Autodesk Inventor part; units mm, degrees
ref_plane "YZ Plane" through (0, 0, 0) normal (1, 0, 0) x (0, 1, 0)
ref_plane "XZ Plane" through (0, 0, 0) normal (0, 1, 0) x (-1, 0, 0)
ref_plane "XY Plane" through (0, 0, 0) normal (0, 0, 1) x (1, 0, 0)
sketch "Эскиз1" plane through (0, 0, 0) normal (0, 0, 1) x (1, 0, 0)
  circle A0 centre (0, 0) radius 10
  line L0 (-3.8095, 3.8095) -> (3.8095, 3.8095)
  line L1 (3.8095, 3.8095) -> (3.8095, -3.8095)
  line L2 (3.8095, -3.8095) -> (-3.8095, -3.8095)
  line L3 (-3.8095, -3.8095) -> (-3.8095, 3.8095)
  line L4 (-3.8095, 3.8095) -> (3.8095, -3.8095) construction
  line L5 (3.8095, 3.8095) -> (-3.8095, -3.8095) construction
  dimension "d0" = 20
extrude "Выдавливание1" add sketch "Эскиз1" along normal blind 36
sketch "Эскиз2" plane through (0, 0, 36) normal (0, 0, 1) x (1, 0, 0)
  line L0 (-3.8095, 3.8095) -> (3.8095, 3.8095)
  circle A0 centre (0, 0) radius 10
  line L1 (9.8151, 1.914) -> (5.5, 1.0725)
  line L2 (5.5, -1.0775) -> (9.8135, -1.9225)
  line L3 (5.5, 0) -> (5.5, 1.0725)
  line L4 (5.5, 1.0725) -> (5.5, -1.0775)
  line L5 (5.587, 8.2937) -> (3.1307, 4.6475)
  line L6 (4.651, 3.1272) -> (8.2986, 5.5797)
  line L7 (3.8891, 3.8891) -> (3.1307, 4.6475)
  line L8 (3.1307, 4.6475) -> (4.651, 3.1272)
  line L9 (-1.914, 9.8151) -> (-1.0725, 5.5)
  line L10 (1.0775, 5.5) -> (1.9225, 9.8135)
  line L11 (0, 5.5) -> (-1.0725, 5.5)
  line L12 (-1.0725, 5.5) -> (1.0775, 5.5)
  line L13 (-8.2937, 5.587) -> (-4.6475, 3.1307)
  line L14 (-3.1272, 4.651) -> (-5.5797, 8.2986)
  line L15 (-3.8891, 3.8891) -> (-4.6475, 3.1307)
  line L16 (-4.6475, 3.1307) -> (-3.1272, 4.651)
  line L17 (-9.8151, -1.914) -> (-5.5, -1.0725)
  line L18 (-5.5, 1.0775) -> (-9.8135, 1.9225)
  line L19 (-5.5, 0) -> (-5.5, -1.0725)
  line L20 (-5.5, -1.0725) -> (-5.5, 1.0775)
  line L21 (-5.587, -8.2937) -> (-3.1307, -4.6475)
  line L22 (-4.651, -3.1272) -> (-8.2986, -5.5797)
  line L23 (-3.8891, -3.8891) -> (-3.1307, -4.6475)
  line L24 (-3.1307, -4.6475) -> (-4.651, -3.1272)
  line L25 (1.914, -9.8151) -> (1.0725, -5.5)
  line L26 (-1.0775, -5.5) -> (-1.9225, -9.8135)
  line L27 (0, -5.5) -> (1.0725, -5.5)
  line L28 (1.0725, -5.5) -> (-1.0775, -5.5)
  line L29 (8.2937, -5.587) -> (4.6475, -3.1307)
  line L30 (3.1272, -4.651) -> (5.5797, -8.2986)
  line L31 (3.8891, -3.8891) -> (4.6475, -3.1307)
  line L32 (4.6475, -3.1307) -> (3.1272, -4.651)
  dimension "d36" = 360
extrude "Выдавливание2" add sketch "Эскиз2" along normal blind 3 contours A0 L2 L4 L3 L1 | L6 L8 L7 L5 A0 | A0 L30 L32 L31 L29 | L10 L12 L11 L9 A0 | A0 L26 L28 L27 L25 | L14 L16 L15 L13 A0 | A0 L22 L24 L23 L21 | L18 L20 L19 L17 A0
chamfer "Фаска1" distance 2 angle 10 1 edges at (4.3588, 6.4706, 39) measured on face at (4.7682, 7.0783, 37)
chamfer "Фаска2" distance 2 angle 10 1 edges at (6.4748, 4.3535, 39) measured on face at (5.8669, 3.9447, 37)
chamfer "Фаска3" distance 2 angle 10 1 edges at (7.6576, 1.4932, 39) measured on face at (8.3768, 1.6335, 37)
chamfer "Фаска4" distance 2 angle 10 1 edges at (7.6567, -1.5, 39) measured on face at (6.9378, -1.3592, 37)
chamfer "Фаска5" distance 2 angle 10 1 edges at (6.4706, -4.3588, 39) measured on face at (7.0783, -4.7682, 37)
chamfer "Фаска6" distance 2 angle 10 1 edges at (4.3535, -6.4748, 39) measured on face at (3.9447, -5.8669, 37)
chamfer "Фаска7" distance 2 angle 10 1 edges at (-1.5, -7.6567, 39) measured on face at (-1.3592, -6.9378, 37)
chamfer "Фаска8" distance 2 angle 10 1 edges at (1.4932, -7.6576, 39) measured on face at (1.6335, -8.3768, 37)
chamfer "Фаска9" distance 2 angle 10 1 edges at (-6.4748, -4.3535, 39) measured on face at (-5.8669, -3.9447, 37)
chamfer "Фаска10" distance 2 angle 10 1 edges at (-4.3588, -6.4706, 39) measured on face at (-4.7682, -7.0783, 37)
chamfer "Фаска11" distance 2 angle 10 1 edges at (-7.6567, 1.5, 39) measured on face at (-6.9378, 1.3592, 37)
chamfer "Фаска12" distance 2 angle 10 1 edges at (-7.6576, -1.4932, 39) measured on face at (-8.3768, -1.6335, 37)
chamfer "Фаска13" distance 2 angle 10 1 edges at (-4.3535, 6.4748, 39) measured on face at (-3.9447, 5.8669, 37)
chamfer "Фаска14" distance 2 angle 10 1 edges at (-6.4706, 4.3588, 39) measured on face at (-7.0783, 4.7682, 37)
chamfer "Фаска15" distance 2 angle 10 1 edges at (1.5, 7.6567, 39) measured on face at (1.3592, 6.9378, 37)
chamfer "Фаска16" distance 2 angle 10 1 edges at (-1.4932, 7.6576, 39) measured on face at (-1.6335, 8.3768, 37)
sketch "Эскиз3" plane through (0, 0, 36) normal (0, 0, 1) x (1, 0, 0)
  point P0 (0, 0)
sketch "Эскиз5" plane through (0, 0, 36) normal (0, 0, 1) x (1, 0, 0)
  point P0 (0, 0)
sketch "Эскиз6" plane through (0, 0, 36) normal (0, 0, 1) x (1, 0, 0)
  line L0 (-1.0725, 5.5) -> (-1.914, 9.8151)
  arc A0 (-1.914, 9.8151) -> (-5.5797, 8.2986) centre (0, 0) ccw
  line L1 (-5.5797, 8.2986) -> (-3.1272, 4.651)
  line L2 (-3.1272, 4.651) -> (-4.6475, 3.1307)
  line L3 (-4.6475, 3.1307) -> (-8.2937, 5.587)
  arc A1 (-8.2937, 5.587) -> (-9.8135, 1.9225) centre (0, 0) ccw
  line L4 (-9.8135, 1.9225) -> (-5.5, 1.0775)
  line L5 (-5.5, 1.0775) -> (-5.5, -1.0725)
  line L6 (-5.5, -1.0725) -> (-9.8151, -1.914)
  arc A2 (-9.8151, -1.914) -> (-8.2986, -5.5797) centre (0, 0) ccw
  line L7 (-8.2986, -5.5797) -> (-4.651, -3.1272)
  line L8 (-4.651, -3.1272) -> (-3.1307, -4.6475)
  line L9 (-3.1307, -4.6475) -> (-5.587, -8.2937)
  arc A3 (-5.587, -8.2937) -> (-1.9225, -9.8135) centre (0, 0) ccw
  line L10 (-1.9225, -9.8135) -> (-1.0775, -5.5)
  line L11 (-1.0775, -5.5) -> (1.0725, -5.5)
  line L12 (1.0725, -5.5) -> (1.914, -9.8151)
  arc A4 (1.914, -9.8151) -> (5.5797, -8.2986) centre (0, 0) ccw
  line L13 (5.5797, -8.2986) -> (3.1272, -4.651)
  line L14 (3.1272, -4.651) -> (4.6475, -3.1307)
  line L15 (4.6475, -3.1307) -> (8.2937, -5.587)
  arc A5 (8.2937, -5.587) -> (9.8135, -1.9225) centre (0, 0) ccw
  line L16 (9.8135, -1.9225) -> (5.5, -1.0775)
  line L17 (5.5, -1.0775) -> (5.5, 1.0725)
  line L18 (5.5, 1.0725) -> (9.8151, 1.914)
  arc A6 (9.8151, 1.914) -> (8.2986, 5.5797) centre (0, 0) ccw
  line L19 (8.2986, 5.5797) -> (4.651, 3.1272)
  line L20 (4.651, 3.1272) -> (3.1307, 4.6475)
  line L21 (3.1307, 4.6475) -> (5.587, 8.2937)
  arc A7 (5.587, 8.2937) -> (1.9225, 9.8135) centre (0, 0) ccw
  line L22 (1.9225, 9.8135) -> (1.0775, 5.5)
  line L23 (1.0775, 5.5) -> (-1.0725, 5.5)
  line L24 (-3.8095, 3.8095) -> (3.8095, 3.8095)
  line L25 (3.8095, 3.8095) -> (3.8095, -3.8095)
  line L26 (3.8095, -3.8095) -> (-3.8095, -3.8095)
  line L27 (-3.8095, -3.8095) -> (-3.8095, 3.8095)
extrude "Выдавливание4" add sketch "Эскиз6" against normal up to surface (36 mm away) contours L24 L25 L26 L27
sketch "Эскиз7" plane through (0, 0, 36) normal (0, 0, 1) x (1, 0, 0)
  line L0 (-5.8493, 2.507) -> (2.507, 5.8493)
  line L1 (2.507, 5.8493) -> (5.8493, -2.507)
  line L2 (5.8493, -2.507) -> (-2.507, -5.8493)
  line L3 (-2.507, -5.8493) -> (-5.8493, 2.507)
  line L4 (-5.8493, 2.507) -> (5.8493, -2.507) construction
  line L5 (2.507, 5.8493) -> (-2.507, -5.8493) construction
  point P0 (0, 0)
  dimension "d95" = 9
  dimension "d96" = 9
extrude "Выдавливание5" cut sketch "Эскиз7" against normal through all
sketch "Эскиз8" plane through (0, 0, 36) normal (0, 0, 1) x (1, 0, 0)
  line L0 (-4.651, -3.1272) -> (-3.1307, -4.6475)
  line L1 (-1.0775, -5.5) -> (1.0725, -5.5)
  line L2 (-3.1307, -4.6475) -> (-1.0775, -5.5)
  line L3 (-1.0775, -5.5) -> (-1.3659, -6.972)
  line L4 (-1.9225, -9.8135) -> (-1.0775, -5.5)
  line L5 (-3.1307, -4.6475) -> (-3.9688, -5.8915)
  line L6 (-3.1307, -4.6475) -> (-5.587, -8.2937)
  line L7 (-3.9688, -5.8915) -> (-1.3659, -6.972)
  line L8 (4.6475, -3.1307) -> (5.8915, -3.9688)
  line L9 (5.5, -1.0775) -> (6.972, -1.3659)
  line L10 (4.6475, -3.1307) -> (5.5, -1.0775)
  line L11 (5.8915, -3.9688) -> (6.972, -1.3659)
  line L12 (3.1307, 4.6475) -> (3.9688, 5.8915)
  line L13 (1.0775, 5.5) -> (1.3659, 6.972)
  line L14 (3.1307, 4.6475) -> (1.0775, 5.5)
  line L15 (3.9688, 5.8915) -> (1.3659, 6.972)
  line L16 (-4.6475, 3.1307) -> (-5.8915, 3.9688)
  line L17 (-5.5, 1.0775) -> (-6.972, 1.3659)
  line L18 (-4.6475, 3.1307) -> (-5.5, 1.0775)
  line L19 (-5.8915, 3.9688) -> (-6.972, 1.3659)
  point P0 (0, 0)
  dimension "d99" = 1.5
  dimension "d100" = 1.5
  dimension "d103" = 360
extrude "Выдавливание6" cut sketch "Эскиз8" against normal through all
sketch "Эскиз9" plane through (0, 0, 36) normal (0, 0, 1) x (1, 0, 0)
  line L0 (-1.3659, -6.972) -> (-1.0775, -5.5)
  line L1 (-1.0775, -5.5) -> (-1, -5)
  line L2 (-3.1307, -4.6475) -> (-3.9688, -5.8915)
  line L3 (-3.1307, -4.6475) -> (-2.4444, -3.6286)
  line L4 (-2.4444, -3.6286) -> (-1, -5)
  line L5 (-3.1307, -4.6475) -> (-1.0775, -5.5)
  line L6 (5.5, -1.0775) -> (5, -1)
  line L7 (4.6475, -3.1307) -> (3.6286, -2.4444)
  line L8 (3.6286, -2.4444) -> (5, -1)
  line L9 (4.6475, -3.1307) -> (5.5, -1.0775)
  line L10 (1.0775, 5.5) -> (1, 5)
  line L11 (3.1307, 4.6475) -> (2.4444, 3.6286)
  line L12 (2.4444, 3.6286) -> (1, 5)
  line L13 (3.1307, 4.6475) -> (1.0775, 5.5)
  line L14 (-5.5, 1.0775) -> (-5, 1)
  line L15 (-4.6475, 3.1307) -> (-3.6286, 2.4444)
  line L16 (-3.6286, 2.4444) -> (-5, 1)
  line L17 (-4.6475, 3.1307) -> (-5.5, 1.0775)
  point P0 (0, 0)
  dimension "d109" = 360
extrude "Выдавливание7" cut sketch "Эскиз9" against normal through all
properties part number "деталь вв"
Check sheet for the modelled part. Datum: model origin and axes. Units: mm. A direction names the side the tool comes from. Round coordinates to 2 decimals unless told otherwise and drop trailing zeros. Order: outer loops, then holes, each group sorted by start corner. A loop starts at its lowest first (then second) coordinate and runs counter-clockwise, first axis right, second up.
(1) Cross-section at C-C, the plane x = -2.5. Enter the section's corners in (y, z).
(2) Cross-section at B-B, the plane x = 0. Enter the section's corners in (y, z), and give its area (3 significant figures).
(3) Scan lines: probe 1 along Y at (x, z) = (8, 36.5); probe 2 along Y at (x, z) = (-2.5, 15); probe 3 along Y at (x, z) = (-3.5, 37). Record each from-to range of solid material in increasing order.
(4) Go/stop test with flat-tipped pins: P1, Ø1.5, axis at y = 7, z = 31.5, coming from the +X side; P2, Ø5, axis at x = -7.5, z = 22.5, coming from the -Y side; P3, Ø8, axis at x = 5, z = 25.5, coming from the -Y side. Record where each tip stops, or that it passes through.
(5) Access from +Z, -Z, +X, -X, +Y, -Y to the whole of each face (thin tool, end or side, straight path). Record for faces 1 (the flat face through (4.47, 6.32, 38.01)), 2 (the flat face through (-3.88, -3.9, 37.48)), 3 (the flat face through (2.686, 6.424, 18.252)).
(6) Cross-section at A-A, the plane z = 23. Enter the section's corners in (x, y).
Check sheet entries:
1. outline: (-9.68, 0) - (-6.5, 0) - (-6.5, 36) - (-9.68, 36) - close; (3.85, 0) - (9.68, 0) - (9.68, 36) - (3.85, 36) - close
2. outline: (-10, 0) - (-4.85, 0) - (-4.85, 36) - (-5.5, 36) - (-5.5, 39) - (-10, 39) - close; (4.85, 0) - (10, 0) - (10, 39) - (5.5, 39) - (5.5, 36) - (4.85, 36) - close
2. area: 398 mm2
3. probe 1: y = -6 to -5.39, -1.57 to 1.56, 5.38 to 6
3. probe 2: y = -9.68 to -6.5, 3.85 to 9.68
3. probe 3: y = -5.2 to -4.28, 4.28 to 5.21
4. P1: stops at x = 7.81
4. P2: stops at y = -8.66
4. P3: stops at y = -9.95
5. face 1: +Z, +Y
5. face 2: +Z
5. face 3: +Z, -Z
6. outline: circle Ø20 at (0, 0); hole (-6.97, 1.37) - (-5.5, 1.08) - (-5.26, 1.04) - (-3.04, -4.51) - (-3.13, -4.65) - (-3.97, -5.89) - (-1.37, -6.97) - (-1.08, -5.5) - (-1.04, -5.26) - (4.51, -3.04) - (4.65, -3.13) - (5.89, -3.97) - (6.97, -1.37) - (5.5, -1.08) - (5.26, -1.04) - (3.04, 4.51) - (3.13, 4.65) - (3.97, 5.89) - (1.37, 6.97) - (1.08, 5.5) - (1.04, 5.26) - (-4.51, 3.04) - (-4.65, 3.13) - (-5.89, 3.97) - close
